Input: part model. Units: mm. Frame: model coordinates. Face numbers are marked on the shaded views. Coordinates: 2 decimals unless noted, no trailing zeros. Write each loop counter-clockwise with the first axis right and the second up, starting at its lowest first coordinate (ties: lowest second). Pieces come first, ordered by that corner, then holes.
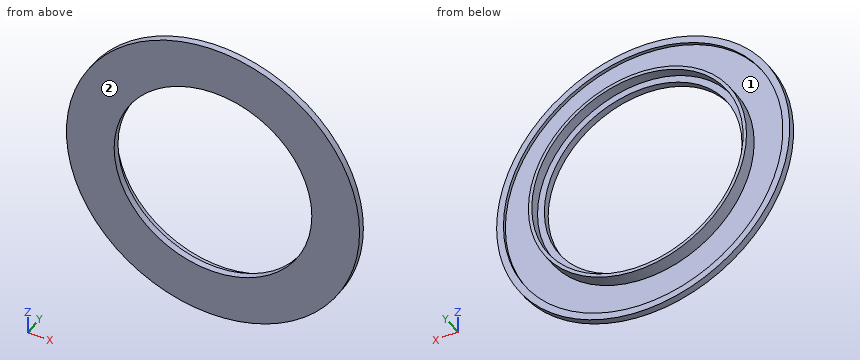
from build123d import *

# Parameters (mm, degrees)
SKETCH1_R           = 43
BOSS_EXTRUDE1_DEPTH = 2
SKETCH2_R           = 41
BOSS_EXTRUDE2_DEPTH = 3
SKETCH3_R           = 30
CUT_EXTRUDE1_DEPTH  = 2
SKETCH4_R           = 28
CUT_EXTRUDE2_DEPTH  = 4
SKETCH5_R           = 41
CUT_EXTRUDE3_DEPTH  = 4
SKETCH6_R           = 32
BOSS_EXTRUDE4_DEPTH = 4
SKETCH7_R           = 31
CUT_EXTRUDE4_DEPTH  = 3
SKETCH8_R           = 29
CUT_EXTRUDE5_DEPTH  = 3


with BuildPart() as part:
    # Sketch1 → Boss-Extrude1 (new body)
    with BuildSketch(Plane(origin=(0, 0, 0), x_dir=(1, 0, 0), z_dir=(0, 1, 0))):
        Circle(SKETCH1_R)
    extrude(amount=BOSS_EXTRUDE1_DEPTH)

    # Sketch2 → Boss-Extrude2 (add)
    with BuildSketch(Plane(origin=(0, 2, 0), x_dir=(1, 0, 0), z_dir=(0, 1, 0))):
        Circle(SKETCH2_R)
    extrude(amount=BOSS_EXTRUDE2_DEPTH)

    # Sketch3 → Cut-Extrude1 (cut)
    with BuildSketch(Plane(origin=(0, 5, 0), x_dir=(1, 0, 0), z_dir=(0, 1, 0))):
        Circle(SKETCH3_R)
    extrude(amount=-CUT_EXTRUDE1_DEPTH, mode=Mode.SUBTRACT)

    # Sketch4 → Cut-Extrude2 (cut, through all)
    with BuildSketch(Plane(origin=(0, 3, 0), x_dir=(1, 0, 0), z_dir=(0, 1, 0))):
        Circle(SKETCH4_R)
    extrude(amount=-CUT_EXTRUDE2_DEPTH, mode=Mode.SUBTRACT)

    # Sketch5 → Cut-Extrude3 (cut)
    with BuildSketch(Plane(origin=(0, 5, 0), x_dir=(1, 0, 0), z_dir=(0, 1, 0))):
        Circle(SKETCH5_R)
    extrude(amount=-CUT_EXTRUDE3_DEPTH, mode=Mode.SUBTRACT)

    # Sketch6 → Boss-Extrude4 (add)
    with BuildSketch(Plane(origin=(0, 1, 0), x_dir=(1, 0, 0), z_dir=(0, 1, 0))):
        Circle(SKETCH6_R)
    extrude(amount=BOSS_EXTRUDE4_DEPTH)

    # Sketch7 → Cut-Extrude4 (cut)
    with BuildSketch(Plane(origin=(0, 5, 0), x_dir=(1, 0, 0), z_dir=(0, 1, 0))):
        Circle(SKETCH7_R)
    extrude(amount=-CUT_EXTRUDE4_DEPTH, mode=Mode.SUBTRACT)

    # Sketch8 → Cut-Extrude5 (cut, through all)
    with BuildSketch(Plane(origin=(0, 2, 0), x_dir=(1, 0, 0), z_dir=(0, 1, 0))):
        Circle(SKETCH8_R)
    extrude(amount=-CUT_EXTRUDE5_DEPTH, mode=Mode.SUBTRACT)


solid = part.part
Item 1: Section query A-A, the plane x = 0. Return loops of the section in (y, z), then the cut area to 3 significant figures.
Item 2: Pull-direction query (X, two-part tool) for the marked faces 1 and 2; classes: released by +X, released by -X, zero draft, split by the parting line, or undercut.
Item 3: Section query C-C, the plane y = 4. Return loops of the section in (x, z).
Item 4: Section query D-D, the plane x = 36.5. Return loops of the section in (y, z), then the cut area to 3 significant figures.
Item 5: Pin query (flat end, axial travel): pin 1 Ø1.5 at (x, y) = (20.5, 4) entering from +Z. Return the tip coordinate at first contact, or that it passes through.
Item 6: Section query B-B, the plane z = 0. Return loops of the section in (x, y), then the cut area to 3 significant figures.
Item 7: Material intervals for line 1 (X direction, y = 1.6, z = 0); line 2 (X direction, y = 0.8, z = 0), sorted ascending.
The answers:
1. outline: (0, -43) - (2, -43) - (2, -41) - (1, -41) - (1, -32) - (5, -32) - (5, -31) - (2, -31) - (2, -29) - (0, -29) - close; (0, 29) - (2, 29) - (2, 31) - (5, 31) - (5, 32) - (1, 32) - (1, 41) - (2, 41) - (2, 43) - (0, 43) - close
1. area: 44.0 mm2
2. face 1: undercut
2. face 2: zero draft
3. outline: circle Ø64 at (0, 0); hole circle Ø62 at (0, 0)
4. outline: (0, -22.73) - (2, -22.73) - (2, -18.67) - (1, -18.67) - (1, 18.67) - (2, 18.67) - (2, 22.73) - (0, 22.73) - close
4. area: 53.6 mm2
5. pin 1: stops at z = 25.18
6. outline: (-43, 0) - (-29, 0) - (-29, 2) - (-31, 2) - (-31, 5) - (-32, 5) - (-32, 1) - (-41, 1) - (-41, 2) - (-43, 2) - close; (29, 0) - (43, 0) - (43, 2) - (41, 2) - (41, 1) - (32, 1) - (32, 5) - (31, 5) - (31, 2) - (29, 2) - close
6. area: 44.0 mm2
7. line 1: x = -43 to -41, -32 to -29, 29 to 32, 41 to 43
7. line 2: x = -43 to -29, 29 to 43
